from build123d import *

# Parameters (mm, degrees)
F0_W         = 104.6088039875
F0_H         = 133.5426568985
F1_DEPTH     = 25.4
F2_T         = -2.54
F3_W         = 19.131584093
F3_H         = 25.4
F4_DEPTH     = 18.1840639561
F5_T         = 2.54
F5_T3_DEPTH  = 27.94
F5_T5_DEPTH  = 133.5426568985
F5_T7_DEPTH  = 104.6088039875
F5_T9_DEPTH  = 54.8444019938
F5_T11_DEPTH = 20.7240639561
F5_T13_DEPTH = 24.211584093
F5_T15_DEPTH = 35.7128179008


# Not quite as in the source:
# - a shell that OpenCascade refuses in one call is made with other operations: the cavity is built on its own and cut out


with BuildPart() as f1:
    # F0 (on Top) → F1 (new body)
    with BuildSketch(Plane.XY):
        with Locations((0, -9.2112720013)):
            Rectangle(F0_W, F0_H)
    extrude(amount=F1_DEPTH)

    # F2
    f2_openings = [f1.faces().sort_by_distance(p)[0] for p in [
        (0, -9.211272, 25.4),
    ]]
    offset(amount=F2_T, openings=f2_openings)

    # F3 (on face) → F4 (join)
    with BuildSketch(Plane.XZ.offset(75.9826004505)):
        with Locations((-9.5657920465, 12.7)):
            Rectangle(F3_W, F3_H)
    extrude(amount=-F4_DEPTH)

    # F5: shell of thickness 2.54, made by hand


with BuildPart() as f5_core1:
    # F5_t2: copy of F1
    add(f1.part)

    # the walls: a layer under each face that stays
    f5_faces = [f5_core1.faces().sort_by_distance(p)[0] for p in [
        (52.3044019938, -9.2112720013, 12.7),
        (-14.9441148554, -66.4438392435, 25.4),
        (49.7644019938, -9.2112720013, 13.97),
        (0, -9.2112720013, 2.54),
        (0, 55.020056448, 13.97),
        (-49.7644019938, -9.2112720013, 13.97),
        (-34.4479930434, -73.4426004505, 13.97),
        (-19.131584093, -65.6205684724, 13.97),
        (-9.5657920465, -57.7985364944, 13.97),
        (0, -65.6205684724, 13.97),
        (24.8822009969, -73.4426004505, 13.97),
        (-52.3044019938, -9.2112720013, 12.7),
        (0, -9.2112720013, 0),
        (0, 57.560056448, 12.7),
    ]]
    thicken(f5_faces, amount=-F5_T, mode=Mode.SUBTRACT)

    # F5_s4 → F5_t3 (cut)
    with BuildSketch(Plane.XY):
        Polygon((49.7390019938, 54.994656448), (52.3044019938, 55.020056448), (52.3044019938, 57.560056448), (49.7644019938, 57.560056448), align=None)
        Polygon((49.7390019938, -73.4172004505), (52.3044019938, -73.4426004505), (52.3044019938, -75.9826004505), (49.7644019938, -75.9826004505), align=None)
        Polygon((-49.7390019938, 54.994656448), (-49.7644019938, 57.560056448), (-52.3044019938, 57.560056448), (-52.3044019938, 55.020056448), align=None)
        Polygon((-49.7390019938, -73.4172004505), (-52.3044019938, -73.4426004505), (-52.3044019938, -75.9826004505), (-49.7644019938, -75.9826004505), align=None)
        Polygon((-19.156984093, -73.4172004505), (-19.131584093, -75.9826004505), (-16.591584093, -75.9826004505), (-16.591584093, -73.4426004505), align=None)
        Polygon((0.0254, -73.4172004505), (-2.54, -73.4426004505), (-2.54, -75.9826004505), (0, -75.9826004505), align=None)
    extrude(amount=F5_T3_DEPTH, mode=Mode.SUBTRACT)

    # F5_s6 → F5_t5 (cut)
    with BuildSketch(Plane.XZ.offset(-57.560056448)):
        Polygon((49.7390019938, 2.5654), (52.3044019938, 2.54), (52.3044019938, 0), (49.7644019938, 0), align=None)
        Polygon((-49.7390019938, 2.5654), (-49.7644019938, 0), (-52.3044019938, 0), (-52.3044019938, 2.54), align=None)
    extrude(amount=F5_T5_DEPTH, mode=Mode.SUBTRACT)

    # F5_s8 → F5_t7 (cut)
    with BuildSketch(Plane.YZ.offset(-52.3044019938)):
        Polygon((54.994656448, 2.5654), (55.020056448, 0), (57.560056448, 0), (57.560056448, 2.54), align=None)
    extrude(amount=F5_T7_DEPTH, mode=Mode.SUBTRACT)

    # F5_s10 → F5_t9 (cut)
    with BuildSketch(Plane.YZ.offset(-2.54)):
        Polygon((-73.4172004505, 2.5654), (-73.4426004505, 0), (-75.9826004505, 0), (-75.9826004505, 2.54), align=None)
    extrude(amount=F5_T9_DEPTH, mode=Mode.SUBTRACT)

    # F5_s12 → F5_t11 (cut)
    with BuildSketch(Plane.XZ.offset(55.2585364944)):
        Polygon((0.0254, 2.5654), (0, 0), (-2.54, 0), (-2.54, 2.54), align=None)
        Polygon((-19.156984093, 2.5654), (-19.131584093, 0), (-16.591584093, 0), (-16.591584093, 2.54), align=None)
    extrude(amount=F5_T11_DEPTH, mode=Mode.SUBTRACT)

    # F5_s14 → F5_t13 (cut)
    with BuildSketch(Plane.YZ.offset(-21.671584093)):
        Polygon((-57.7731364944, 2.5654), (-57.7985364944, 0), (-60.3385364944, 0), (-60.3385364944, 2.54), align=None)
    extrude(amount=F5_T13_DEPTH, mode=Mode.SUBTRACT)

    # F5_s16 → F5_t15 (cut)
    with BuildSketch(Plane.YZ.offset(-52.3044019938)):
        Polygon((-73.4172004505, 2.5654), (-73.4426004505, 0), (-75.9826004505, 0), (-75.9826004505, 2.54), align=None)
    extrude(amount=F5_T15_DEPTH, mode=Mode.SUBTRACT)


with BuildPart() as f1_1:
    add(f1.part)

    # what is left inside the walls is the cavity
    f5_cavity = [f5_core1.part.solids().sort_by_distance(p)[0] for p in [
        (-2.5654, -65.553224, 12.7),
    ]]
    add(f5_cavity, mode=Mode.SUBTRACT)


solid = f1_1.part
Source: CAD feature listing. Evaluate the final solid. Frame: model axes, mm. A direction names the side the tool comes from. Give positions to 0.01 mm unless a question says otherwise; leave off trailing zeros. Order: outer loops, then holes, each group sorted by start corner. A loop starts at its lowest first (then second) coordinate and runs counter-clockwise, first axis right, second up. Notation, with made-up numbers: (50.5, 35) -> (60.5, 35) arc R15 ccw to (60.5, 42) -> close; hole circle Ø2 at (78, 5). An arc over 180 degrees is marked (long way). Write item = value, one per line.
Q1. Pull-direction query (X, two-part tool) for faces 1 (the face through (-1, -75.983, 13)), 2 (the face through (-52.304, -10, 13)), 3 (the face through (-10, -68, 2.54)); classes: released by +X, released by -X, zero draft, split by the parting line, or undercut.
Data:
face_1 = zero draft
face_2 = released by -X
face_3 = undercut
Q2. Cut plane B-B, the plane z = 11. Output: boundary loops of the cut face in (x, y).
Data:
outline = (-52.3, -75.98) -> (-16.59, -75.98) -> (-16.59, -60.34) -> (-2.54, -60.34) -> (-2.54, -75.98) -> (52.3, -75.98) -> (52.3, 57.56) -> (-52.3, 57.56) -> close; hole (-49.76, -73.44) -> (-19.13, -73.44) -> (-19.13, -57.8) -> (0, -57.8) -> (0, -73.44) -> (49.76, -73.44) -> (49.76, 55.02) -> (-49.76, 55.02) -> close
Q3. Set-up query: faces 4 (the face through (-10, -68, 22.86)), 5 (the face through (25, -73.443, 14)), 6 (the face through (-1, -10, 0)). Return all of +Z, -Z, +X, -X, +Y, -Y with unobstructed straight access to the full face (end or side cutting, diameter ignored); none if empty.
Data:
face_4 = -Y
face_5 = +Z
face_6 = -Z, +X, -X, +Y, -Y
Q4. Cut plane C-C, the plane y = -20. Output: boundary loops of the cut face in (x, z), and give its area (3 significant figures).
Data:
outline = (-52.3, 0) -> (52.3, 0) -> (52.3, 25.4) -> (49.76, 25.4) -> (49.76, 2.54) -> (-49.76, 2.54) -> (-49.76, 25.4) -> (-52.3, 25.4) -> close
area = 382 mm^2
Q5. Cut plane A-A, the plane x = 17.5. Output: boundary loops of the cut face in (y, z), and give its area (3 significant figures).
Data:
outline = (-75.98, 0) -> (57.56, 0) -> (57.56, 25.4) -> (55.02, 25.4) -> (55.02, 2.54) -> (-73.44, 2.54) -> (-73.44, 25.4) -> (-75.98, 25.4) -> close
area = 455 mm^2
Q6. Pin query (flat end, axial travel): pin 1 (11 mm diameter, centred on x = -10.5, z = 15.5, fed in from -Y); pin 2 (6 mm diameter, centred on x = -10, y = 13.5, fed in from +Z). Return the tip coordinate at first contact, or that it passes through.
Data:
pin_1 = -60.34
pin_2 = 2.54
Q7. Material intervals for line 1 (X direction, y = -62, z = 20.5); line 2 (Y direction, x = 39, z = 22.5); line 3 (X direction, y = -16.5, z = 17.5), sorted ascending. Write a range as from..to.
Data:
line_1 = -52.3..-49.76, -19.13..-16.59, -2.54..0, 49.76..52.3
line_2 = -75.98..-73.44, 55.02..57.56
line_3 = -52.3..-49.76, 49.76..52.3
